```python
from build123d import *

# Parameters (mm, degrees)
F1_DEPTH = 4.064
F2_DEPTH = 9.525
F3_R     = 3.81


with BuildPart() as f1:
    # F0 (on Top) → F1 (new body)
    with BuildSketch(Plane.XY):
        with BuildLine():
            Line((-8.128, 0), (-10.795, 0))
            ThreePointArc((-10.795, 0), (0, -10.795), (10.795, 0))
            Line((10.795, 0), (8.128, 0))
            ThreePointArc((8.128, 0), (0, -8.128), (-8.128, 0))
        make_face()
        with BuildLine():
            ThreePointArc((0, 10.795), (-7.633218, 7.633218), (-10.795, 0))
            Line((-10.795, 0), (-8.128, 0))
            ThreePointArc((-8.128, 0), (0, 8.128), (8.128, 0))
            Line((8.128, 0), (10.795, 0))
            ThreePointArc((10.795, 0), (7.633218, 7.633218), (0, 10.795))
        make_face()
        with BuildLine():
            Line((-10.795, 7.62), (-10.795, 0))
            ThreePointArc((-10.795, 0), (-7.633218, 7.633218), (0, 10.795))
            Line((0, 10.795), (-7.62, 10.795))
            ThreePointArc((-7.62, 10.795), (-9.865064, 9.865064), (-10.795, 7.62))
        make_face()
        with BuildLine():
            ThreePointArc((0, 10.795), (7.633218, 7.633218), (10.795, 0))
            Line((10.795, 0), (10.795, 7.62))
            ThreePointArc((10.795, 7.62), (9.865064, 9.865064), (7.62, 10.795))
            Line((7.62, 10.795), (0, 10.795))
        make_face()
    extrude(amount=F1_DEPTH)

    # F0 (on Top) → F2 (join)
    with BuildSketch(Plane.XY):
        with BuildLine():
            ThreePointArc((8.128, 0), (0, 8.128), (-8.128, 0))
            Line((-8.128, 0), (-3.175, 0))
            ThreePointArc((-3.175, 0), (0, 3.175), (3.175, 0))
            Line((3.175, 0), (8.128, 0))
        make_face()
        with BuildLine():
            Line((-3.175, 0), (-8.128, 0))
            ThreePointArc((-8.128, 0), (0, -8.128), (8.128, 0))
            Line((8.128, 0), (3.175, 0))
            ThreePointArc((3.175, 0), (0, -3.175), (-3.175, 0))
        make_face()
    extrude(amount=F2_DEPTH)

    # F3
    f3_edges = [f1.edges().sort_by_distance(p)[0] for p in [
        (-3.175, 0, 9.525),
    ]]
    fillet(f3_edges, radius=F3_R)


solid = f1.part
```
Verification items for the finished model (mm, model axes). A direction names the side the tool comes from. Give positions to 0.01 mm unless a question says otherwise; leave off trailing zeros. Order: outer loops, then holes, each group sorted by start corner. A loop starts at its lowest first (then second) coordinate and runs counter-clockwise, first axis right, second up. Notation, with made-up numbers: (0, 79.5) -> (23, 79.5) arc R13 cw to (23, 89.5) -> close; hole circle Ø5 at (-37, -11.5). An arc over 180 degrees is marked (long way). Use a Markdown table: item, result.
1) Mould release check, pull along Y, two halves, no side actions. Record for faces 3 (the cylindrical face through (1.762, 7.935, 6.756)), 4 (the cylindrical face through (3.03, -0.95, 2.82)), 5 (the flat face through (4, 6, 9.525)): pulls with the +Y half, pulls with the -Y half, needs draft (parallel to the pull), parting line crosses it, or undercut.
Results:
| item | result |
|---|---|
| face 3 | parting line crosses it |
| face 4 | undercut |
| face 5 | needs draft |
2) Depth check by flat-ended pin: pin 1 Ø1.5 at (x, z) = (7.5, 5) entering from -Y; pin 2 Ø4 at (x, z) = (0, 8.5) entering from +Y; pin 3 Ø1 at (y, z) = (-1, 3.5) entering from -X. Enter the tip coordinate at first touch or a pass-through.
Results:
| item | result |
|---|---|
| pin 1 | y = -4.53 |
| pin 2 | y = 8.13 |
| pin 3 | x = -10.78 |
3) Tool access check on faces 1 (the flat face through (-10.795, 4, 2)), 2 (the flat face through (5, 7, 4.064)). Record the directions out of +Z, -Z, +X, -X, +Y, -Y that give a thin tool (end or side, any length) a straight path to the whole face; none if there is none.
Results:
| item | result |
|---|---|
| face 1 | +Z, -Z, -X, +Y, -Y |
| face 2 | +Z |
4) Section check A-A, the plane x = 0. Record the boundary of the cut face in (y, z) (3 decimals).
Results:
| item | result |
|---|---|
| outline | (-10.795, 0) -> (-3.175, 0) -> (-3.175, 5.715) arc R3.81 ccw to (-6.985, 9.525) -> (-8.128, 9.525) -> (-8.128, 4.064) -> (-10.795, 4.064) -> close; (3.175, 0) -> (10.795, 0) -> (10.795, 4.064) -> (8.128, 4.064) -> (8.128, 9.525) -> (6.985, 9.525) arc R3.81 ccw to (3.175, 5.715) -> close |
5) Material ranges on probe 1 along Y at (x, z) = (0, 1.5) (3 decimals); probe 2 along Y at (x, z) = (0, 4.1) (3 decimals), recorded low to high.
Results:
| item | result |
|---|---|
| probe 1 | -10.795 to -3.175, 3.175 to 10.795 |
| probe 2 | -8.128 to -3.175, 3.175 to 8.128 |
6) Section check D-D, the plane x = -9.5. Record the boundary of the cut face in (y, z), then the cut area to 3 significant figures.
Results:
| item | result |
|---|---|
| outline | (-5.13, 0) -> (10.18, 0) -> (10.18, 4.06) -> (-5.13, 4.06) -> close |
| area | 62.2 mm² |
7) Section check C-C, the plane z = 5.25. Record the boundary of the cut face in (x, y) (3 decimals), then the cut area to 3 significant figures.
Results:
| item | result |
|---|---|
| outline | circle Ø16.256 at (0, 0); hole circle Ø6.35 at (0, 0) |
| area | 176 mm² |
8) Section check B-B, the plane z = 1. Record the boundary of the cut face in (x, y) (3 decimals).
Results:
| item | result |
|---|---|
| outline | (-10.795, 0) arc R10.795 ccw to (10.795, 0) -> (10.795, 7.62) arc R3.175 ccw to (7.62, 10.795) -> (-7.62, 10.795) arc R3.175 ccw to (-10.795, 7.62) -> close; hole circle Ø6.35 at (0, 0) |
